from build123d import *

# Parameters (mm, degrees)
SKETCH5_R           = 3.175
BOSS_EXTRUDE3_DEPTH = 35.814
CHAMFER1_SIZE       = 0.680357143
BOSS_EXTRUDE4_DEPTH = 4.3688
SKETCH8_OUTSIDE_W   = 167.676
SKETCH8_OUTSIDE_H   = 169.404
SKETCH8_OUTSIDE_R   = 5.588
CUT_EXTRUDE3_DEPTH  = 42.079404635
CUT_EXTRUDE3_DRAFT  = -60


with BuildPart() as part:
    # Sketch5 → Boss-Extrude3 (new body)
    with BuildSketch(Plane(origin=(20.0914, 0, 0), x_dir=(0, 0, -1), z_dir=(1, 0, 0))):
        Circle(SKETCH5_R)
    extrude(amount=-BOSS_EXTRUDE3_DEPTH)

    # Chamfer1
    chamfer1_edges = [part.edges().sort_by_distance(p)[0] for p in [
        (20.0914, 0, 3.175),
    ]]
    chamfer(chamfer1_edges, length=CHAMFER1_SIZE)

    # Sketch6 → Boss-Extrude4 (add)
    with BuildSketch(Plane.ZY.offset(15.7226)):
        Polygon((5.588, 3.226233304), (0, 6.452466608), (-5.588, 3.226233304), (-5.588, -3.226233304), (0, -6.452466608), (5.588, -3.226233304), align=None)
    extrude(amount=BOSS_EXTRUDE4_DEPTH)


with BuildPart() as cut_extrude3_tool:
    # Sketch8 outside → Cut-Extrude3 (with draft: the straight prism first)
    with BuildSketch(Plane.ZY.offset(20.0914)):
        Rectangle(SKETCH8_OUTSIDE_W, SKETCH8_OUTSIDE_H)
        Circle(SKETCH8_OUTSIDE_R, mode=Mode.SUBTRACT)
    extrude(amount=-CUT_EXTRUDE3_DEPTH)
    # Cut-Extrude3: the draft: its side faces are tilted about the plane it starts from
    cut_extrude3_sides = [cut_extrude3_tool.faces().sort_by_distance(p)[0] for p in [
        (0.948302318, -84.702, 0),
        (0.948302318, 0, 83.838),
        (0.948302318, 84.702, 0),
        (0.948302318, 0, -83.838),
        (0.948302318, 0, -5.588),
    ]]
    draft(cut_extrude3_sides, Plane.ZY.offset(20.0914), CUT_EXTRUDE3_DRAFT)


with BuildPart() as part_1:
    add(part.part)

    # Cut-Extrude3: cut by cut_extrude3_tool
    add(cut_extrude3_tool.part, mode=Mode.SUBTRACT)


solid = part_1.part
The model under review builds one solid part; all positions refer to its coordinate system, in mm. A direction names the side the tool comes from. Round coordinates to 2 decimals unless told otherwise and drop trailing zeros. Order: outer loops, then holes, each group sorted by start corner. A loop starts at its lowest first (then second) coordinate and runs counter-clockwise, first axis right, second up. Notation, with made-up numbers: (54, 88.25) -> (71, 88.25) arc R15 ccw to (71, 111.25) -> close; hole circle Ø11 at (57, 51.25). An arc over 180 degrees is marked (long way). Return JSON: item names as keys, results as strings.
1. The part is to be moulded in two halves that separate along X. For faces 3 (the face through (20.091, 0, 0)), 4 (the face through (-17.88, 4.82, 2.83)), 5 (the face through (-19.972, -2.909, 5.011)), say which applies: +X half, -X half, draft (parallel to the pull), parting line (faces both ways), or undercut.
Answer block:
{"face 3": "+X half", "face 4": "draft", "face 5": "-X half"}
2. Insertion check: P1, Ø1, axis at x = -2, y = 3, coming from the -Z side; P2, Ø3, axis at x = 14, y = -1.5, coming from the +Z side (3 decimals); P3, Ø2, axis at x = 15.5, z = 0.5, coming from the +Y side (3 decimals); P4, Ø2, axis at x = 4, z = -4.5, coming from the +Y side. Each pin has a flat end and moves straight along its axis. Give the tip position at first contact, or say it passes through.
Answer block:
{"P1": "stops at z = -1.96", "P2": "stops at z = 3.175", "P3": "stops at y = 3.175", "P4": "passes through"}
3. For L1, parallel to X at y = -3.5, z = 2.5; L2, parallel to Y at x = 16.5, z = 1.5, list the stretches that pass through material, from the lowest coordinate up. Write a range as [from, to].
Answer block:
{"L1": "x = [-20.09, -15.72]", "L2": "y = [-2.8, 2.8]"}
4. Take a section at A-A (x = -0.5). Write out the cut boundary in (y, z) (3 decimals).
Answer block:
{"outline": "circle Ø6.35 at (0, 0)"}
5. For faces 1 (the face through (-19.972, 5.794, 0.014)), 2 (the face through (-15.723, -3, -3)), list the 3-axis set-ups (+Z, -Z, +X, -X, +Y, -Y) from which the entire face can be reached by the end or side of a thin tool; tool diameter is ignored.
Answer block:
{"face 1": "-X, +Y", "face 2": "+X"}
